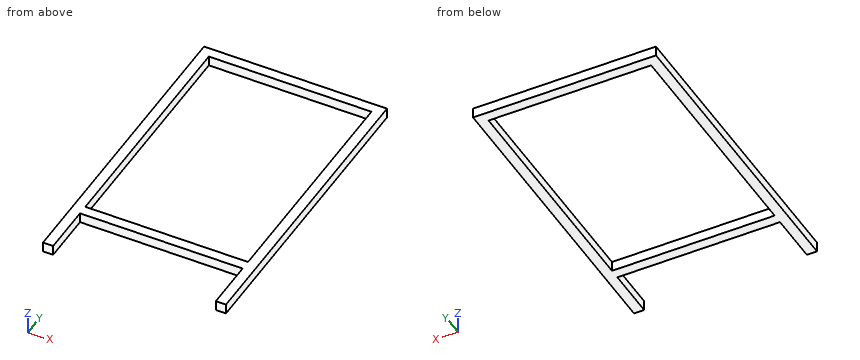
from build123d import *

# Parameters (mm, degrees)
SKETCH1_W           = 320
SKETCH1_H           = 460
BOSS_EXTRUDE1_DEPTH = 10


with BuildPart() as part:
    # Sketch1 → Boss-Extrude1 (new, symmetric)
    with BuildSketch(Plane.XY):
        Polygon((-180, -600), (-180, 0), (180, 0), (180, -600), (160, -600), (160, -500), (-160, -500), (-160, -600), align=None)
        with Locations((0, -250)):
            Rectangle(SKETCH1_W, SKETCH1_H, mode=Mode.SUBTRACT)
    extrude(amount=BOSS_EXTRUDE1_DEPTH, both=True)


solid = part.part
The listing builds one solid part. Answer for the finished solid, in the listing's coordinates (mm). Coordinates: 2 decimals unless noted, no trailing zeros. Loops run counter-clockwise (first coordinate to the right, second up) from the corner with the lowest first, then second, coordinate; pieces in that order, holes last. Notation, with made-up numbers: (70, -3) -> (118, -3) arc R25 ccw to (118, 14) -> close; hole circle Ø1 at (19.25, -26.5). An arc over 180 degrees is marked (long way). Answer in a Markdown table with one row per item. Add a question column.
1. A flat-ended cylindrical pin translates along its axis: P1, Ø1.5, axis at x = -4, z = -4, coming from the -Y side. Find the tip coordinate at first contact, or state that the pin passes through.
2. The part is cut by section C-C, the plane y = -551.5. Write down the section's boundary in (x, z).
3. The part is cut by section A-A, the plane x = 5.5. Write down the section's boundary in (y, z).
4. Consider line 1 (Y direction, x = 34.5, z = 7.5); line 2 (X direction, y = -420, z = -6.25). Determine where each line is inside the solid, lowest interval first. Write a range as [from, to].
5. The part is cut by section B-B, the plane z = 2. Write down the section's boundary in (x, y), then the cut area to 3 significant figures.
Answer below:
| question | item | result |
|---|---|---|
| 1 | P1 | y = -500 |
| 2 | outline | (-180, -10) -> (-160, -10) -> (-160, 10) -> (-180, 10) -> close; (160, -10) -> (180, -10) -> (180, 10) -> (160, 10) -> close |
| 3 | outline | (-500, -10) -> (-480, -10) -> (-480, 10) -> (-500, 10) -> close; (-20, -10) -> (0, -10) -> (0, 10) -> (-20, 10) -> close |
| 4 | line 1 | [-500, -480], [-20, 0] |
| 4 | line 2 | [-180, -160], [160, 180] |
| 5 | outline | (-180, -600) -> (-160, -600) -> (-160, -500) -> (160, -500) -> (160, -600) -> (180, -600) -> (180, 0) -> (-180, 0) -> close; hole (-160, -480) -> (160, -480) -> (160, -20) -> (-160, -20) -> close |
| 5 | area | 36,800 mm2 |
